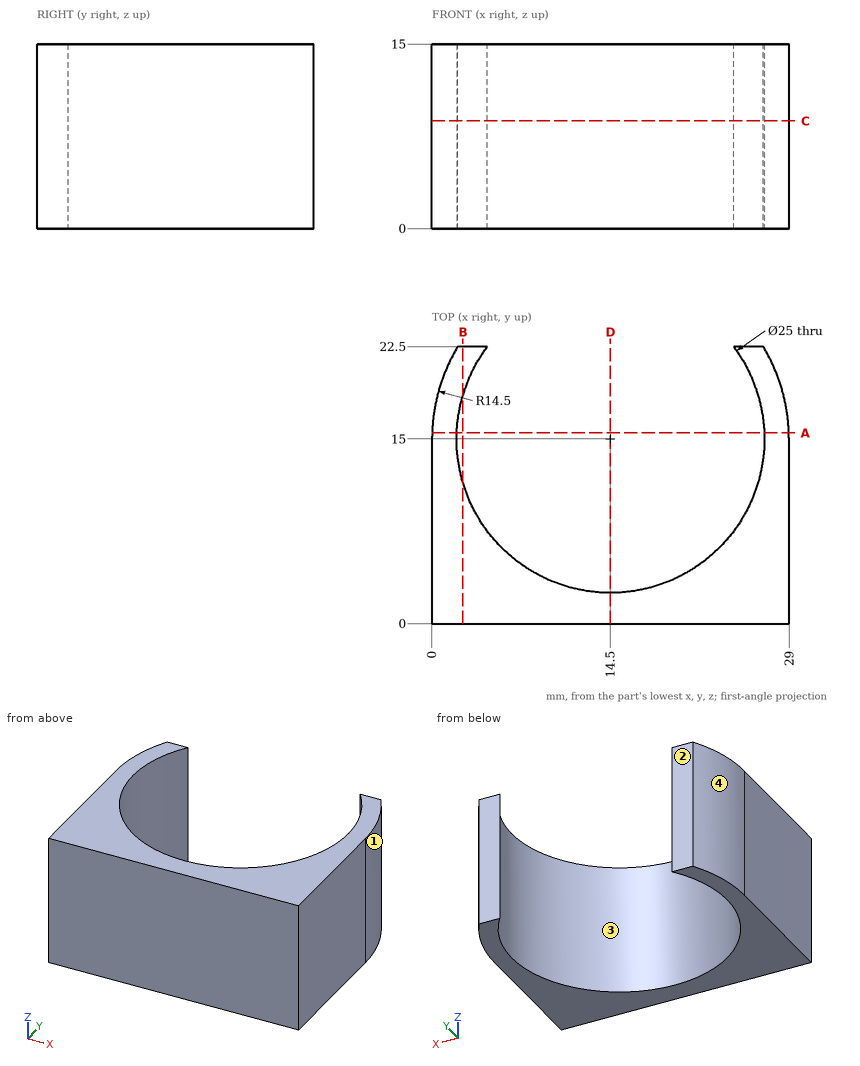
The figure shows three views and two pictorial views of one solid part (mm, origin at its lowest corner). Answer the questions. Coordinates: 2 decimals unless noted, no trailing zeros. Loops run counter-clockwise (first coordinate to the right, second up) from the corner with the lowest first, then second, coordinate; pieces in that order, holes last. Notation, with made-up numbers: (30, 25) -> (43, 25) arc R28 ccw to (43, 64) -> close; hole circle Ø7 at (-38, -38.75). An arc over 180 degrees is marked (long way). Use one line per item in the form item = value. Start each with the question number.
Item 1: The part is cut by section C-C on z = 8.75. Determine the outline of the cut face in (x, y).
Item 2: Flat-ended cylindrical pins translate along their axes: pin 1 Ø4 at (y, z) = (20, 5) entering from -X; pin 2 Ø6 at (x, z) = (10.5, 4) entering from +Y; pin 3 Ø8 at (x, z) = (19.5, 9.5) entering from +Y. Find the tip coordinate at first contact, or state that the pin passes through.
Item 3: Consider L1, parallel to X at y = 13.5, z = 3.5; L2, parallel to X at y = 15, z = 2.75; L3, parallel to Y at x = 3.5, z = 9.5. Determine where each line is inside the solid, lowest interval first. Write a range as [from, to].
Item 4: The part is cut by section B-B on x = 2.5. Determine the outline of the cut face in (y, z).
Item 5: The part is cut by section A-A on y = 15.5. Determine the outline of the cut face in (x, z), then the cut area to 3 significant figures.
Item 6: The mould has two halves that part along X. Classify the marked faces 1, 2, 3 and 4: released by +X, released by -X, zero draft, split by the parting line, or undercut.
Item 7: The part is cut by section D-D on x = 14.5. Determine the outline of the cut face in (y, z), then the cut area to 3 significant figures.
Answer key:
q1.outline = (0, 0) -> (29, 0) -> (29, 15) arc R14.5 ccw to (26.91, 22.5) -> (24.5, 22.5) arc R12.5 cw (long way) to (4.5, 22.5) -> (2.09, 22.5) arc R14.5 ccw to (0, 15) -> close
q2.pin_1 = 0.31
q2.pin_2 = 4.64
q2.pin_3 = 6.33
q3.L1 = [0, 2.09], [26.91, 29]
q3.L2 = [0, 2], [27, 29]
q3.L3 = [0, 9.06], [20.94, 22.5]
q4.outline = (0, 0) -> (11.5, 0) -> (11.5, 15) -> (0, 15) -> close; (18.5, 0) -> (22.5, 0) -> (22.5, 15) -> (18.5, 15) -> close
q5.outline = (0.01, 0) -> (2.01, 0) -> (2.01, 15) -> (0.01, 15) -> close; (26.99, 0) -> (28.99, 0) -> (28.99, 15) -> (26.99, 15) -> close
q5.area = 60.0 mm2
q6.face_1 = released by +X
q6.face_2 = zero draft
q6.face_3 = undercut
q6.face_4 = released by -X
q7.outline = (0, 0) -> (2.5, 0) -> (2.5, 15) -> (0, 15) -> close
q7.area = 37.5 mm2
